from build123d import *

# Parameters (mm, degrees)
F0_W     = 860
F0_H     = 700
F1_DEPTH = 20
F2_R     = 5
F3_DEPTH = 20.001
F4_R     = 9.5
F5_DEPTH = 20.001
F6_R     = 10


with BuildPart() as f1:
    # F0 (on Front) → F1 (new body)
    with BuildSketch(Plane.XZ):
        Rectangle(F0_W, F0_H)
    extrude(amount=F1_DEPTH)

    # F2 (on face) → F3 (cut, through all)
    with BuildSketch(Plane.XZ.offset(20)):
        with Locations((390, 0)):
            Circle(F2_R)
    extrude(amount=-F3_DEPTH, mode=Mode.SUBTRACT)

    # F4 (on face) → F5 (cut, through all)
    with BuildSketch(Plane.XZ.offset(20)):
        with Locations((390, -45)):
            Circle(F4_R)
    extrude(amount=-F5_DEPTH, mode=Mode.SUBTRACT)

    # F6
    f6_edges = [f1.edges().sort_by_distance(p)[0] for p in [
        (430, -10, 350),
        (430, -10, -350),
        (-430, -10, 350),
        (-430, -10, -350),
    ]]
    fillet(f6_edges, radius=F6_R)


solid = f1.part
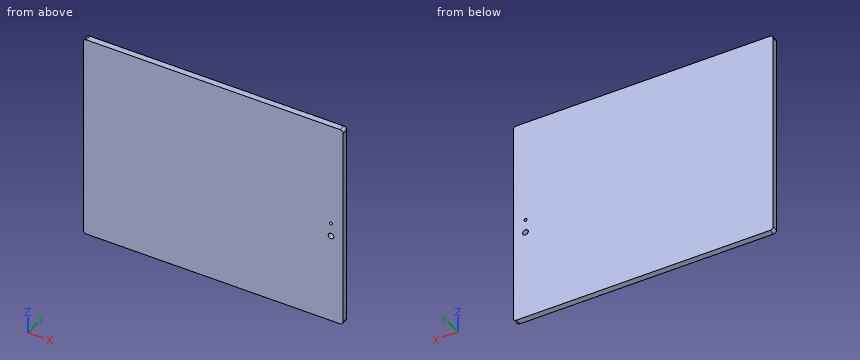
Part model, mm, in its own coordinate system. Coordinates: 2 decimals unless noted, no trailing zeros. Loops run counter-clockwise (first coordinate to the right, second up) from the corner with the lowest first, then second, coordinate; pieces in that order, holes last. Notation, with made-up numbers: M 45,35 L 100,35 A19 cw 100,48 Z; hole C -29,-4 d4. An arc over 180 degrees is marked long. Use a Markdown table: item, result. Add a question column.
Q1. Probe L1, parallel to Z at x = 390, y = -6.5; L2, parallel to X at y = -15.25, z = -3.5. List the from-to ranges inside material, lowest first.
Q2. Pin check, flat tip, straight feed: P1, Ø11.5, axis at x = 390, z = 0, coming from the +Y side. Stop position of the tip, or through.
Q3. Cut at A-A (z = -45). Write the cut outline in (x, y), and give its area (3 significant figures).
Worked out:
| question | item | result |
|---|---|---|
| 1 | L1 | z = -350 to -54.5, -35.5 to -5, 5 to 350 |
| 1 | L2 | x = -430 to 386.43, 393.57 to 430 |
| 2 | P1 | stops at y = 0 |
| 3 | outline | M -430,-20 L 380.5,-20 L 380.5,0 L -430,0 Z; M 399.5,-20 L 430,-20 L 430,0 L 399.5,0 Z |
| 3 | area | 16,800 mm2 |
